Design review of the part built by this model. Coordinates are the model's own, in mm. A direction names the side the tool comes from. Coordinates: 2 decimals unless noted, no trailing zeros. Order: outer loops, then holes, each group sorted by start corner. A loop starts at its lowest first (then second) coordinate and runs counter-clockwise, first axis right, second up. Notation, with made-up numbers: (-26, 3) -> (-18, 3) arc R27 ccw to (-18, 37) -> close; hole circle Ø7 at (66, 64.5). An arc over 180 degrees is marked (long way). Write item = value, one per line.
```python
from build123d import *

# Parameters (mm, degrees)
SKETCH2_W           = 25
SKETCH2_H           = 10
BOSS_EXTRUDE1_DEPTH = 40
SKETCH3_W           = 10.4
SKETCH3_H           = 35
CUT_EXTRUDE1_DEPTH  = 44.084219849
SKETCH4_W           = 18
SKETCH4_H           = 6.8
CUT_EXTRUDE2_DEPTH  = 5
CUT_EXTRUDE3_DEPTH  = 30


with BuildPart() as part:
    # Sketch2 → Boss-Extrude1 (new body)
    with BuildSketch(Plane.XY):
        Rectangle(SKETCH2_W, SKETCH2_H)
    extrude(amount=BOSS_EXTRUDE1_DEPTH)

    # Sketch3 → Cut-Extrude1 (cut, through all)
    with BuildSketch(Plane(origin=(0, 5, 0), x_dir=(1, 0, 0), z_dir=(0, 1, 0))):
        with Locations((0, -22.5)):
            Rectangle(SKETCH3_W, SKETCH3_H)
    extrude(amount=-CUT_EXTRUDE1_DEPTH, mode=Mode.SUBTRACT)

    # Sketch4 → Cut-Extrude2 (cut)
    with BuildSketch(Plane(origin=(0, 5, 0), x_dir=(1, 0, 0), z_dir=(0, 1, 0))):
        with Locations((0, -10.4)):
            Rectangle(SKETCH4_W, SKETCH4_H)
    extrude(amount=-CUT_EXTRUDE2_DEPTH, mode=Mode.SUBTRACT)

    # Sketch5 → Cut-Extrude3 (cut)
    with BuildSketch(Plane.XY.offset(7)):
        Polygon((5.2, 3.8), (9, 0), (5.2, -3.8), align=None)
        Polygon((-5.2, -3.8), (-5.2, 3.8), (-9, 0), align=None)
    extrude(amount=CUT_EXTRUDE3_DEPTH, mode=Mode.SUBTRACT)


solid = part.part
```
(1) For L1, parallel to X at y = 4, z = 29.5; L2, parallel to Z at x = 6.25, y = 0.25; L3, parallel to Z at x = 5, y = 2.75, list the stretches that pass through material, from the lowest coordinate up.
Report:
L1 = -12.5 to -5.2, 5.2 to 12.5
L2 = 0 to 7, 37 to 40
L3 = 0 to 5
(2) Insertion check: pin 1 (1.9 mm diameter, centred on x = 7, y = 1.5, fed in from -Z); pin 2 (5 mm diameter, centred on x = -2, y = -1.5, fed in from +Z). Each pin has a flat end and moves straight along its axis. Give the tip position at first contact, or say it passes through.
Report:
pin_1 = 0
pin_2 = 5
(3) We need section D-D (z = 37.5). Write out the cut boundary in (x, y).
Report:
outline = (-12.5, -5) -> (-5.2, -5) -> (-5.2, 5) -> (-12.5, 5) -> close; (5.2, -5) -> (12.5, -5) -> (12.5, 5) -> (5.2, 5) -> close
(4) We need section B-B (x = 7.75). Write out the cut boundary in (y, z).
Report:
outline = (-5, 0) -> (5, 0) -> (5, 7) -> (-1.25, 7) -> (-1.25, 37) -> (1.25, 37) -> (1.25, 13.8) -> (5, 13.8) -> (5, 40) -> (-5, 40) -> close
(5) We need section A-A (z = 17). Write out the cut boundary in (x, y).
Report:
outline = (-12.5, -5) -> (-5.2, -5) -> (-5.2, -3.8) -> (-9, 0) -> (-5.2, 3.8) -> (-5.2, 5) -> (-12.5, 5) -> close; (5.2, -5) -> (12.5, -5) -> (12.5, 5) -> (5.2, 5) -> (5.2, 3.8) -> (9, 0) -> (5.2, -3.8) -> close
(6) We need section C-C (y = 2.5). Write out the cut boundary in (x, z), and give its area (3 significant figures).
Report:
outline = (-12.5, 0) -> (12.5, 0) -> (12.5, 40) -> (5.2, 40) -> (5.2, 37) -> (6.5, 37) -> (6.5, 13.8) -> (9, 13.8) -> (9, 7) -> (5.2, 7) -> (5.2, 5) -> (-5.2, 5) -> (-5.2, 7) -> (-9, 7) -> (-9, 13.8) -> (-6.5, 13.8) -> (-6.5, 37) -> (-5.2, 37) -> (-5.2, 40) -> (-12.5, 40) -> close
area = 524 mm²
(7) The part is to be moulded in two halves that separate along X. For faces 5 (the flat face through (12.5, 0, 20)), 6 (the flat face through (5.2, -4, 26)), 7 (the flat face through (9, 0, 40)), 8 (the flat face through (-12.5, 0, 20)), say which applies: released by +X, released by -X, zero draft, split by the parting line, or undercut.
Report:
face_5 = released by +X
face_6 = undercut
face_7 = zero draft
face_8 = released by -X
(8) For faces 1 (the flat face through (0, 0, 5)), 2 (the flat face through (7, -2, 22)), 3 (the flat face through (-7, 2, 7)), 4 (the flat face through (5.4, 5, 19.7)), list the 3-axis set-ups (+Z, -Z, +X, -X, +Y, -Y) from which the entire face can be reached by the end or side of a thin tool; tool diameter is ignored.
Report:
face_1 = +Z, +Y, -Y
face_2 = none
face_3 = +Y
face_4 = +Z, -Z, +X, -X, +Y
